```python
from build123d import *

# Parameters (mm, degrees)
SKETCH_W     = 9.5
SKETCH_H     = 6
SKETCH_W_2   = 1.65
SKETCH_H_2   = 1.35
PAD_DEPTH    = 1
SKETCH001_W  = 5.5
SKETCH001_H  = 4
PAD001_DEPTH = 4
SKETCH002_W  = 1.65
SKETCH002_H  = 1.35
POCKET_DEPTH = 2
PAD002_DEPTH = 4


with BuildPart() as part:
    # Sketch → Pad (new body)
    with BuildSketch(Plane.XY):
        Rectangle(SKETCH_W, SKETCH_H)
        with Locations((1.425, 0)):
            Rectangle(SKETCH_W_2, SKETCH_H_2, mode=Mode.SUBTRACT)
    extrude(amount=PAD_DEPTH)

    # Sketch001 (on Face10 of Pad) → Pad001 (join)
    with BuildSketch(Plane.XY.offset(1)):
        Rectangle(SKETCH001_W, SKETCH001_H)
    extrude(amount=PAD001_DEPTH)

    # Sketch002 (on Face4 of Pad001) → Pocket (cut)
    with BuildSketch(Plane(origin=(0, 0, 0), x_dir=(1, 0, 0), z_dir=(0, 0, -1))):
        with Locations((1.425, 0)):
            Rectangle(SKETCH002_W, SKETCH002_H)
    extrude(amount=-POCKET_DEPTH, mode=Mode.SUBTRACT)

    # Sketch003 (on Face11 of Pocket) → Pad002 (join)
    with BuildSketch(Plane(origin=(0, 2, 0), x_dir=(-1, 0, 0), z_dir=(0, 1, 0))):
        Polygon((-2.75, 5), (-2.40625, 5.363092), (-2.0625, 5), (-1.71875, 5.363092), (-1.375, 5), (-1.03125, 5.363092), (-0.6875, 5), (-0.34375, 5.363092), (0, 5), (0.34375, 5.363092), (0.6875, 5), (1.03125, 5.363092), (1.375, 5), (1.71875, 5.363092), (2.0625, 5), (2.40625, 5.363092), (2.75, 5), (2.760715, 4.584067), (-2.75, 4.584067), align=None)
    extrude(amount=-PAD002_DEPTH)


solid = part.part
```
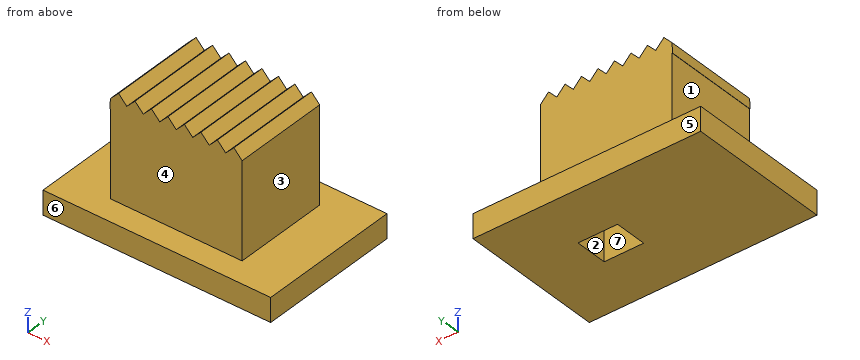
The listing builds one solid part. Answer for the finished solid, in the listing's coordinates (mm). Face numbers are marked on the shaded views. A direction names the side the tool comes from. Coordinates: 2 decimals unless noted, no trailing zeros. Write each loop counter-clockwise with the first axis right and the second up, starting at its lowest first coordinate (ties: lowest second). Pieces come first, ordered by that corner, then holes. Notation, with made-up numbers: (1.25, 30) - (47.25, 30) arc R21 ccw to (47.25, 63) - close; hole circle Ø2 at (56.25, 76.5). An arc over 180 degrees is marked (long way). Return JSON: item names as keys, results as strings. Group by question number.
1. A cutting plane is placed at C-C, the plane x = -1.25. Determine the outline of the cut face in (y, z), plus the area to 3 significant figures.
2. Determine the mould class of the marked faces 5, 6 and 7 for opening direction Y: released by +Y, released by -Y, zero draft, split by the parting line, or undercut.
3. A cutting plane is placed at D-D, the plane z = 1.25. Determine the outline of the cut face in (x, y) (3 decimals).
4. Which of the six approach directions +Z, -Z, +X, -X, +Y, -Y give full straight-line access (tool end or side, diameter ignored) to the marked faces 1, 2, 3 and 4?
5. Given pin 1 (3 mm diameter, centred on y = -0.5, z = 3.5, fed in from -X); pin 2 (2 mm diameter, centred on x = -1.5, z = 4.5, fed in from -Y); pin 3 (1.3 mm diameter, centred on x = -1.5, z = 2.5, fed in from +Y), each flat-ended and moving along its own axis, determine where each tip first touches the part or whether it passes through.
6. Straight lines are drawn through the part: L1, parallel to Y at x = 0.75, z = 1.3 (3 decimals); L2, parallel to Y at x = 1, z = 0.95 (3 decimals); L3, parallel to X at y = -0.2, z = 0.4. For each, find the intervals that lie inside material, in ascending order.
7. A cutting plane is placed at A-A, the plane z = 0.4. Determine the outline of the cut face in (x, y) (3 decimals), plus the area to 3 significant figures.
Ans:
{
 "1": {"outline": "(-3, 0) - (3, 0) - (3, 1) - (2, 1) - (2, 5.13) - (-2, 5.13) - (-2, 1) - (-3, 1) - close", "area": "22.5 mm²"},
 "2": {"face 5": "released by +Y", "face 6": "released by -Y", "face 7": "undercut"},
 "3": {"outline": "(-2.75, -2) - (2.75, -2) - (2.75, 2) - (-2.75, 2) - close; hole (0.6, -0.675) - (2.25, -0.675) - (2.25, 0.675) - (0.6, 0.675) - close"},
 "4": {"face 1": "-X, +Y, -Y", "face 2": "-Z", "face 3": "+Z, +X, +Y, -Y", "face 4": "+Z, +X, -X, -Y"},
 "5": {"pin 1": "x = -2.76", "pin 2": "y = -2", "pin 3": "y = 2"},
 "6": {"L1": "-2 to -0.675, 0.675 to 2", "L2": "-3 to -0.675, 0.675 to 3", "L3": "-4.75 to 0.6, 2.25 to 4.75"},
 "7": {"outline": "(-4.75, -3) - (4.75, -3) - (4.75, 3) - (-4.75, 3) - close; hole (0.6, -0.675) - (2.25, -0.675) - (2.25, 0.675) - (0.6, 0.675) - close", "area": "54.8 mm²"}
}
